Verification items for the finished model (mm, model axes). Face numbers are marked on the shaded views. A direction names the side the tool comes from. Give positions to 0.01 mm unless a question says otherwise; leave off trailing zeros. Write each loop counter-clockwise with the first axis right and the second up, starting at its lowest first coordinate (ties: lowest second). Pieces come first, ordered by that corner, then holes.
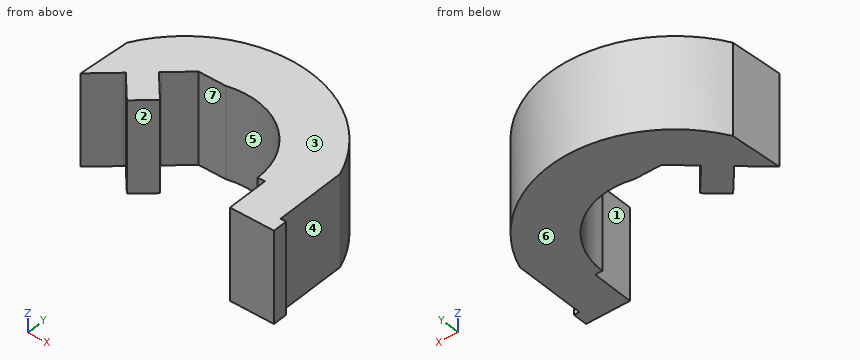
from build123d import *

# Parameters (mm, degrees)
BOSS_EXTRUDE1_DEPTH = 12.7


with BuildPart() as part:
    # Sketch3 → Boss-Extrude1 (new body)
    with BuildSketch(Plane.XY):
        with BuildLine():
            Line((-39.908456621, 10.757671301), (-40.099131524, 10.589864623))
            Line((-40.099131524, 10.589864623), (-43.499378585, 7.5974196))
            Line((-43.499378585, 7.5974196), (-43.044803336, 14.723327074))
            ThreePointArc((-43.044803336, 14.723327074), (-26.54219977, 23.502903952), (-11.60681582, 12.262298946))
            Line((-11.60681582, 12.262298946), (-11.60681582, 5.15464013))
            Line((-11.60681582, 5.15464013), (-11.60681582, 2.440752288))
            Line((-11.60681582, 2.440752288), (-10.85681582, 2.440752288))
            Line((-10.85681582, 2.440752288), (-10.85681582, 0.448752288))
            Line((-10.85681582, 0.448752288), (-16.916890922, 0.448752288))
            Line((-16.916890922, 0.448752288), (-16.916890922, 6.194752288))
            Line((-16.916890922, 6.194752288), (-17.900227072, 6.194752288))
            ThreePointArc((-17.900227072, 6.194752288), (-21.783197569, 14.066907933), (-30.379177034, 15.843824196))
            Line((-30.379177034, 15.843824196), (-34.129177034, 15.843824196))
            Line((-34.129177034, 15.843824196), (-37.088703748, 13.23924258))
            Line((-37.088703748, 13.23924258), (-37.279378651, 13.071435901))
            Line((-37.279378651, 13.071435901), (-34.203525113, 9.576413645))
            Line((-34.203525113, 9.576413645), (-36.832603083, 7.262649045))
            Line((-36.832603083, 7.262649045), (-39.908456621, 10.757671301))
        make_face()
    extrude(amount=-BOSS_EXTRUDE1_DEPTH)


solid = part.part
Item 1: Release check for a two-part mould opening along X. For the marked faces 4, 5, 6 and 7 record: released by +X, released by -X, zero draft, split by the parting line, or undercut.
Answer key:
face 4: released by +X
face 5: undercut
face 6: zero draft
face 7: undercut
Item 2: Sectioned sample at C-C on y = 3.75. Record the cut outline in (x, z), then the cut area to 3 significant figures.
Answer key:
outline: (-16.92, -12.7) - (-11.61, -12.7) - (-11.61, 0) - (-16.92, 0) - close
area: 67.4 mm2
Item 3: Sectioned sample at D-D on x = -13. Record the cut outline in (y, z), then the cut area to 3 significant figures.
Answer key:
outline: (0.45, -12.7) - (15.14, -12.7) - (15.14, 0) - (0.45, 0) - close
area: 187 mm2
Item 4: Sectioned sample at B-B on z = -11.5. Record the cut outline in (x, y), then the cut area to 3 significant figures.
Answer key:
outline: (-43.5, 7.6) - (-39.91, 10.76) - (-36.83, 7.26) - (-34.2, 9.58) - (-37.28, 13.07) - (-34.13, 15.84) - (-30.38, 15.84) arc R10 cw to (-17.9, 6.19) - (-16.92, 6.19) - (-16.92, 0.45) - (-10.86, 0.45) - (-10.86, 2.44) - (-11.61, 2.44) - (-11.61, 12.26) arc R17.4 ccw to (-43.04, 14.72) - close
area: 317 mm2
Item 5: Depth check by flat-ended pin: pin 1 (1.1 mm diameter, centred on x = -32.5, z = -4.5, fed in from -Y); pin 2 (3 mm diameter, centred on y = 17, z = -7, fed in from -X); pin 3 (3 mm diameter, centred on y = 20, z = -2.5, fed in from +X); pin 4 (4 mm diameter, centred on y = 9, z = -1.5, fed in from -X). Enter the tip coordinate at first touch or a pass-through.
Answer key:
pin 1: stops at y = 15.84
pin 2: stops at x = -42.58
pin 3: stops at x = -15.64
pin 4: stops at x = -43.5
Item 6: Set-up check for the marked faces 1, 2 and 3: record each of +Z, -Z, +X, -X, +Y, -Y from which the full face is reachable in a straight line by a thin tool's end or side.
Answer key:
face 1: +Z, -Z, -X, -Y
face 2: +Z, -Z, -Y
face 3: +Z, +X, -X, +Y, -Y
Item 7: Scan lines: line 1 along X through (y, z) = (9.25, -4.5); line 2 along X through (y, z) = (7.5, -9.75); line 3 along X through (y, z) = (1.5, -7.5). Record each from-to range of solid material in increasing order.
Answer key:
line 1: x = -43.39 to -41.62, -38.58 to -34.57, -18.39 to -11.61
line 2: x = -37.04 to -36.56, -17.99 to -11.61
line 3: x = -16.92 to -10.86
Item 8: Sectioned sample at A-A on x = -36. Record the cut outline in (y, z).
Answer key:
outline: (8, -12.7) - (11.62, -12.7) - (11.62, 0) - (8, 0) - close; (14.2, -12.7) - (21.56, -12.7) - (21.56, 0) - (14.2, 0) - close
